Work out the finished part from the listing and answer in its coordinate system (mm). Face numbers are marked on the shaded views. A direction names the side the tool comes from. Round coordinates to 2 decimals unless told otherwise and drop trailing zeros. Loops run counter-clockwise (first coordinate to the right, second up) from the corner with the lowest first, then second, coordinate; pieces in that order, holes last. Notation, with made-up numbers: (40.5, 47) - (58.5, 47) arc R32 ccw to (58.5, 85) - close; hole circle Ø9 at (73, 19). An arc over 180 degrees is marked (long way). Return JSON: item names as keys, results as strings.
from build123d import *

# Parameters (mm, degrees)
SKETCH_8_W          = 150
SKETCH_8_H          = 200
EXTRUDE_3_DEPTH     = 230
SHELL_2_T           = 2.5
CUT_EXTRUDE_3_DEPTH = 5
SKETCH_11_W         = 142.5
SKETCH_11_H         = 22.5
CUT_EXTRUDE_4_DEPTH = 5


with BuildPart() as part:
    # 草图8 → 凸台-拉伸3 (new body)
    with BuildSketch(Plane(origin=(0, -2.5, 0), x_dir=(-1, 0, 0), z_dir=(0, -1, 0))):
        with Locations((-277.189390083, -102.212193571)):
            Rectangle(SKETCH_8_W, SKETCH_8_H)
    extrude(amount=-EXTRUDE_3_DEPTH)

    # 抽壳2
    shell_2_openings = [part.faces().sort_by_distance(p)[0] for p in [
        (202.189390083, 112.5, 102.212193571),
        (277.189390083, 227.5, 102.212193571),
    ]]
    offset(amount=SHELL_2_T, openings=shell_2_openings, kind=Kind.INTERSECTION)

    # 草图10 → 切除-拉伸3 (cut)
    with BuildSketch(Plane.XY.offset(204.712193571)):
        Polygon((354.689390083, 23), (324.689390083, 23), (324.689390083, 203), (202.189390083, 203), (202.189390083, 23), (202.189390083, 20), (354.689390083, 20), align=None)
    extrude(amount=-CUT_EXTRUDE_3_DEPTH, mode=Mode.SUBTRACT)

    # 草图11 → 切除-拉伸4 (cut)
    with BuildSketch(Plane.XY.offset(204.712193571)):
        with Locations((273.439390083, 8.75)):
            Rectangle(SKETCH_11_W, SKETCH_11_H)
    extrude(amount=-CUT_EXTRUDE_4_DEPTH, mode=Mode.SUBTRACT)


solid = part.part
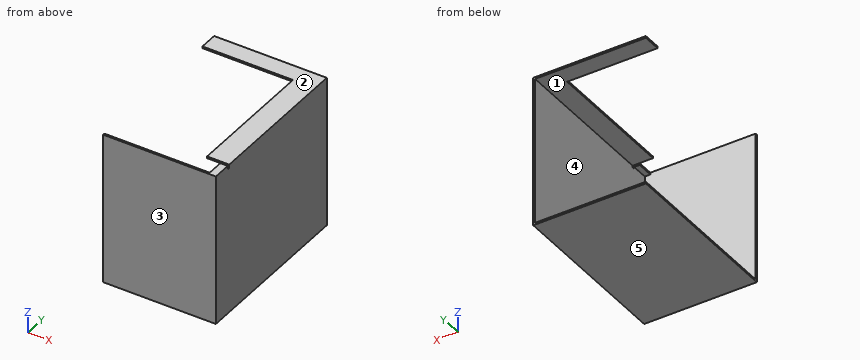
1) A tool of negligible diameter and unlimited length cuts with its end or side. For the marked faces 4 and 5, from which of +Z, -Z, +X, -X, +Y, -Y can it reach the whole face along a straight path? Write none if from no direction.
Verdict:
{"face 4": "-X, +Y", "face 5": "-Z, +X, -X, +Y, -Y"}
2) Find the intervals of material crossed by L1, parallel to Z at x = 336, y = 205; L2, parallel to Z at x = 301, y = 172; L3, parallel to X at y = 213, z = 150, in increasing order.
Verdict:
{"L1": "z = -0.29 to 2.21, 202.21 to 204.71", "L2": "z = -0.29 to 2.21", "L3": "x = 352.19 to 354.69"}
3) Section A-A (x = 312) is taken. Give the vertices of the cut face in (y, z), and give its area (3 significant figures).
Verdict:
{"outline": "(-5, -0.29) - (227.5, -0.29) - (227.5, 2.21) - (-2.5, 2.21) - (-2.5, 204.71) - (-5, 204.71) - close; (203, 202.21) - (227.5, 202.21) - (227.5, 204.71) - (203, 204.71) - close", "area": "1,150 mm2"}
4) Determine the mould class of the marked faces 1, 2 and 3 for opening direction Z: pulls with the +Z half, pulls with the -Z half, needs draft (parallel to the pull), parting line crosses it, or undercut.
Verdict:
{"face 1": "undercut", "face 2": "pulls with the +Z half", "face 3": "needs draft"}
5) Flat-ended cylindrical pins translate along their axes: pin 1 (4 mm diameter, centred on x = 306, y = 68.5, fed in from +Z); pin 2 (10 mm diameter, centred on y = 39.5, z = 155, fed in from -X); pin 3 (1.2 mm diameter, centred on x = 354, y = 21, fed in from +Z). Find the tip coordinate at first contact, or state that the pin passes through.
Verdict:
{"pin 1": "stops at z = 2.21", "pin 2": "stops at x = 352.19", "pin 3": "stops at z = 199.71"}
6) Section B-B (y = 63) is taken. Give the vertices of the cut face in (x, z), and give its area (3 significant figures).
Verdict:
{"outline": "(202.19, -0.29) - (354.69, -0.29) - (354.69, 204.71) - (324.69, 204.71) - (324.69, 202.21) - (352.19, 202.21) - (352.19, 2.21) - (202.19, 2.21) - close", "area": "956 mm2"}
7) Section C-C (z = 189) is taken. Give the vertices of the cut face in (x, y).
Verdict:
{"outline": "(202.19, -5) - (354.69, -5) - (354.69, 227.5) - (352.19, 227.5) - (352.19, -2.5) - (202.19, -2.5) - close"}
